For this review, take the finished solid that the model builds, in its own axes (mm). A direction names the side the tool comes from. Give positions to 0.01 mm unless a question says otherwise; leave off trailing zeros. Loops run counter-clockwise (first coordinate to the right, second up) from the corner with the lowest first, then second, coordinate; pieces in that order, holes last.
```python
from build123d import *

# Parameters (mm, degrees)
BOSS_EXTRU_1_DEPTH      = 30
ENL_V_MAT_EXTRU_1_DEPTH = 11


with BuildPart() as part:
    # Esquisse1 → Boss.-Extru.1 (new body)
    with BuildSketch(Plane.XY):
        Polygon((-8.475934619, -4.771699816), (-8.475934619, -2.271699816), (-5.496550637, -2.271699816), (-5.496550637, 0.228300184), (-2.517166656, 0.228300184), (-2.517166656, 2.728300184), (0.462833344, 2.728300184), (0.462833344, 5.228300184), (-49.537166656, 5.228300184), (-49.537166656, -4.771699816), align=None)
    extrude(amount=BOSS_EXTRU_1_DEPTH)

    # Esquisse2 → Enlèv. mat.-Extru.1 (cut, through all)
    with BuildSketch(Plane.XZ.offset(4.771699816)):
        with BuildLine():
            Line((-167.240462798, 10), (-49.537166656, 10))
            Line((-49.537166656, 10), (-19.537166656, 10))
            ThreePointArc((-19.537166656, 10), (-14.537166656, 15), (-19.537166656, 20))
            Line((-19.537166656, 20), (-49.537166656, 20))
            Line((-49.537166656, 20), (-167.240462798, 20))
            Line((-167.240462798, 20), (-402.647055084, 20))
            Line((-402.647055084, 20), (-402.647055084, 10))
            Line((-402.647055084, 10), (-167.240462798, 10))
        make_face()
    extrude(amount=-ENL_V_MAT_EXTRU_1_DEPTH, mode=Mode.SUBTRACT)


solid = part.part
```
Item 1: Take a section at D-D on y = 3.75. Give the boundary of the cut face in (x, z).
Answer:
outline: (-49.54, 0) - (0.46, 0) - (0.46, 30) - (-49.54, 30) - (-49.54, 20) - (-19.54, 20) arc R5 cw to (-19.54, 10) - (-49.54, 10) - close
Item 2: Clearance check with flat-ended pins moving along their axes: pin 1 Ø5 at (y, z) = (-1, 22) entering from +X; pin 2 Ø2.5 at (x, z) = (-1, 15) entering from -Y; pin 3 Ø6 at (x, z) = (-34, 11) entering from -Y; pin 4 Ø3.5 at (x, z) = (-6.5, 15) entering from -Y. State where each tip first meets the part, or that it passes through.
Answer:
pin 1: stops at x = -2.52
pin 2: stops at y = 2.73
pin 3: stops at y = -4.77
pin 4: stops at y = -2.27
Item 3: The part is to be moulded in two halves that separate along Z. For faces 1 (the flat face through (-7, -2.272, 15)), 2 (the flat face through (-25, 0, 0)), 3 (the flat face through (-34, 0, 20)), 4 (the cylindrical face through (-14.54, 0.16, 14.89)), say which applies: released by +Z, released by -Z, zero draft, split by the parting line, or undercut.
Answer:
face 1: zero draft
face 2: released by -Z
face 3: undercut
face 4: undercut
Item 4: For L1, parallel to Z at x = -45, y = 0.75; L2, parallel to X at y = 1.5, z = 20.5; L3, parallel to Y at x = -3, z = 9.25, list the stretches that pass through material, from the lowest coordinate up.
Answer:
L1: z = 0 to 10, 20 to 30
L2: x = -49.54 to -2.52
L3: y = 0.23 to 5.23
Item 5: Take a section at C-C on y = 0.75. Give the boundary of the cut face in (x, z).
Answer:
outline: (-49.54, 0) - (-2.52, 0) - (-2.52, 30) - (-49.54, 30) - (-49.54, 20) - (-19.54, 20) arc R5 cw to (-19.54, 10) - (-49.54, 10) - close
Item 6: Take a section at B-B on z = 15. Give the boundary of the cut face in (x, y), and give its area (3 significant figures).
Answer:
outline: (-14.54, -4.77) - (-8.48, -4.77) - (-8.48, -2.27) - (-5.5, -2.27) - (-5.5, 0.23) - (-2.52, 0.23) - (-2.52, 2.73) - (0.46, 2.73) - (0.46, 5.23) - (-14.54, 5.23) - close
area: 105 mm2
Item 7: Take a section at A-A on x = -32.5. Give the boundary of the cut face in (y, z).
Answer:
outline: (-4.77, 0) - (5.23, 0) - (5.23, 10) - (-4.77, 10) - close; (-4.77, 20) - (5.23, 20) - (5.23, 30) - (-4.77, 30) - close
Item 8: Tool access review of faces 5 (the flat face through (-8.476, -4, 15)), 6 (the flat face through (-29, -4.772, 21)), 7 (the flat face through (-35, 0, 10)): name each direction out of +Z, -Z, +X, -X, +Y, -Y from which nothing blocks a thin tool from reaching the whole face with its end or side.
Answer:
face 5: +Z, -Z, +X, -Y
face 6: +Z, -Z, +X, -X, -Y
face 7: -X, +Y, -Y
